Check sheet for the modelled part. Datum: model origin and axes. Units: mm. Give positions to 0.01 mm unless a question says otherwise; leave off trailing zeros. Write each loop counter-clockwise with the first axis right and the second up, starting at its lowest first coordinate (ties: lowest second). Pieces come first, ordered by that corner, then holes. Notation, with made-up numbers: M 4,78 L 16,78 A13 ccw 16,95 Z; hole C -6,-32.5 d6. An arc over 180 degrees is marked long. Use CSV: the item, a comma, the result in double quotes. Start each with the question number.
1. Depth check by flat-ended pin: P1, Ø3, axis at x = 12.5, z = -17.5, coming from the -Y side; P2, Ø1.5, axis at y = 1, z = -26.5, coming from the -X side. Enter the tip coordinate at first touch or a pass-through.
2. Cross-section at C-C, the plane z = -19.5. Enter the section's corners in (x, y), and give its area (3 significant figures).
3. Cross-section at B-B, the plane y = 1.1. Enter the section's corners in (x, z).
4. Cross-section at A-A, the plane x = 12.5. Enter the section's corners in (y, z).
5. Scan lines: line 1 (Z direction, x = 12.5, y = 2.05); line 2 (X direction, y = 2.35, z = -17.5); line 3 (Z direction, x = 12, y = 1.2). Record each from-to range of solid material in increasing order.
6. Mould release check, pull along X, two halves, no side actions. Record for faces 1 (the face through (0, 1, -17)), 2 (the face through (14, 1.5, -15.5)), 3 (the face through (9.5, 0, -17.7)): +X half, -X half, draft (parallel to the pull), parting line (faces both ways), or undercut.
from build123d import *

# Parameters (mm, degrees)
SKETCH1_W           = 25
SKETCH1_H           = 35
BOSS_EXTRUDE1_DEPTH = 3
SKETCH2_R           = 2.5
CUT_EXTRUDE1_DEPTH  = 12


with BuildPart() as part:
    # Sketch1 → Boss-Extrude1 (new body)
    with BuildSketch(Plane(origin=(0, 0, 0), x_dir=(1, 0, 0), z_dir=(0, 1, 0))):
        with Locations((12.5, 17.5)):
            Rectangle(SKETCH1_W, SKETCH1_H)
    extrude(amount=BOSS_EXTRUDE1_DEPTH)

    # Sketch2 → Cut-Extrude1 (cut)
    with BuildSketch(Plane(origin=(0, 0, 0), x_dir=(1, 0, 0), z_dir=(0, 1, 0))):
        with Locations(Location((12.5, 17.5, 0), (0, 0, 90))):
            Circle(SKETCH2_R)
    extrude(amount=CUT_EXTRUDE1_DEPTH, mode=Mode.SUBTRACT)


solid = part.part
Worked answers:
1,P1,"passes through"
1,P2,"stops at x = 0"
2,outline,"M 0,0 L 11,0 L 11,3 L 0,3 Z; M 14,0 L 25,0 L 25,3 L 14,3 Z"
2,area,"66.0 mm^2"
3,outline,"M 0,-35 L 25,-35 L 25,0 L 0,0 Z; hole C 12.5,-17.5 d5"
4,outline,"M 0,-35 L 3,-35 L 3,-20 L 0,-20 Z; M 0,-15 L 3,-15 L 3,0 L 0,0 Z"
5,line 1,"z = -35 to -20, -15 to 0"
5,line 2,"x = 0 to 10, 15 to 25"
5,line 3,"z = -35 to -19.95, -15.05 to 0"
6,face 1,"-X half"
6,face 2,"undercut"
6,face 3,"draft"
